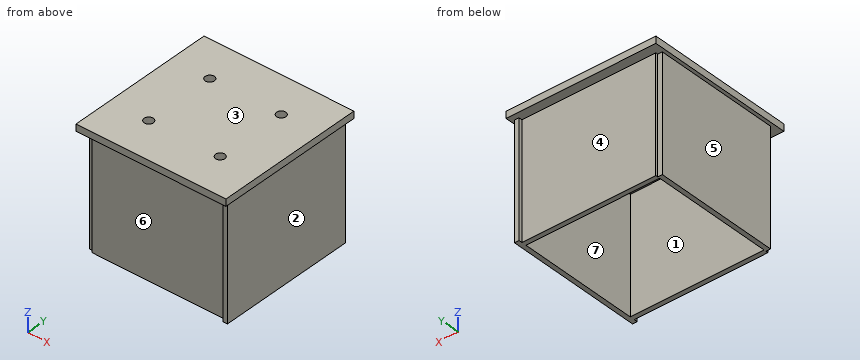
```python
from build123d import *

# Parameters (mm, degrees)
SKETCH1_W           = 65
SKETCH1_H           = 65
SKETCH1_R           = 2
BOSS_EXTRUDE1_DEPTH = 3
SKETCH4_W           = 2
SKETCH4_H           = 60
SKETCH4_H_2         = 55
BOSS_EXTRUDE3_DEPTH = 50


with BuildPart() as part:
    # Sketch1 → Boss-Extrude1 (new body)
    with BuildSketch(Plane.XY):
        Rectangle(SKETCH1_W, SKETCH1_H)
        with Locations((-15.5, 15.5)):
            Circle(SKETCH1_R, mode=Mode.SUBTRACT)
        with Locations((15.5, 15.5)):
            Circle(SKETCH1_R, mode=Mode.SUBTRACT)
        with Locations((15.5, -15.5)):
            Circle(SKETCH1_R, mode=Mode.SUBTRACT)
        with Locations((-15.5, -15.5)):
            Circle(SKETCH1_R, mode=Mode.SUBTRACT)
    extrude(amount=BOSS_EXTRUDE1_DEPTH)

    # Sketch4 → Boss-Extrude3 (add)
    with BuildSketch(Plane(origin=(0, 0, 0), x_dir=(-1, 0, 0), z_dir=(0, 0, -1))):
        with Locations((-30, 0)):
            Rectangle(SKETCH4_W, SKETCH4_H)
        Polygon((29, -26.5), (-29, -26.5), (-29, -28.5), (29, -28.5), (29, -27.5), align=None)
        with Locations((30, 0)):
            Rectangle(SKETCH4_W, SKETCH4_H_2)
        Polygon((29, 27.5), (29, 28.5), (-29, 28.5), (-29, 26.5), (29, 26.5), align=None)
    extrude(amount=BOSS_EXTRUDE3_DEPTH)


solid = part.part
```
The model under review builds one solid part; all positions refer to its coordinate system, in mm. Face numbers are marked on the shaded views. A direction names the side the tool comes from. Round coordinates to 2 decimals unless told otherwise and drop trailing zeros. Order: outer loops, then holes, each group sorted by start corner. A loop starts at its lowest first (then second) coordinate and runs counter-clockwise, first axis right, second up. Notation, with made-up numbers: (32, -25.75) -> (85, -25.75) arc R28 ccw to (85, 6.25) -> close; hole circle Ø3 at (71.5, 26.5). An arc over 180 degrees is marked (long way). One line per item, written item: value. Start each with the question number.
Q1. Take a section at D-D (x = -6). Write out the cut boundary in (y, z), and give its area (3 significant figures).
Q2. Take a section at C-C (z = -32.5). Write out the cut boundary in (x, y).
Q3. Wall thickness on line 1 (Y direction, x = 15.5, z = 2.25); line 2 (X direction, y = 15, z = 1); line 3 (X direction, y = 7, z = -25): over which ranges is each line inside the solid? List them lowest first.
Q4. Take a section at B-B (y = 15.5). Write out the cut boundary in (x, z).
Q5. Clearance check with flat-ended pins moving along their axes: pin 1 Ø5 at (y, z) = (-0.5, -15.5) entering from -X; pin 2 Ø15 at (x, z) = (-12, -32.5) entering from +Y; pin 3 Ø8 at (x, z) = (1, -22.5) entering from -Y; pin 4 Ø5 at (x, y) = (-15.5, -15.5) entering from +Z. State where each tip first meets the part, or that it passes through.
Q6. Machinability: for the marked faces 1, 2, 3 and 4, which of the approach directions +Z, -Z, +X, -X, +Y, -Y give a long, thin tool a straight path to every point of the face, cutting with its end or side? Answer none if there is none.
Q7. Take a section at A-A (x = 15.5). Write out the cut boundary in (y, z), and give its area (3 significant figures).
Q8. Mouldability with a two-part tool opening along X and no side actions: class the marked faces 5, 6 and 7 as released by +X, released by -X, zero draft, split by the parting line, or undercut.
Reported:
1. outline: (-32.5, 0) -> (-28.5, 0) -> (-28.5, -50) -> (-26.5, -50) -> (-26.5, 0) -> (26.5, 0) -> (26.5, -50) -> (28.5, -50) -> (28.5, 0) -> (32.5, 0) -> (32.5, 3) -> (-32.5, 3) -> close
1. area: 395 mm2
2. outline: (-31, -27.5) -> (-29, -27.5) -> (-29, -28.5) -> (29, -28.5) -> (29, -30) -> (31, -30) -> (31, 30) -> (29, 30) -> (29, 28.5) -> (-29, 28.5) -> (-29, 27.5) -> (-31, 27.5) -> close; hole (-29, -26.5) -> (29, -26.5) -> (29, 26.5) -> (-29, 26.5) -> close
3. line 1: y = -32.5 to -17.5, -13.5 to 13.5, 17.5 to 32.5
3. line 2: x = -32.5 to -17.44, -13.56 to 13.56, 17.44 to 32.5
3. line 3: x = -31 to -29, 29 to 31
4. outline: (-32.5, 0) -> (-31, 0) -> (-31, -50) -> (-29, -50) -> (-29, 0) -> (-17.5, 0) -> (-17.5, 3) -> (-32.5, 3) -> close; (-13.5, 0) -> (13.5, 0) -> (13.5, 3) -> (-13.5, 3) -> close; (17.5, 0) -> (29, 0) -> (29, -50) -> (31, -50) -> (31, 0) -> (32.5, 0) -> (32.5, 3) -> (17.5, 3) -> close
5. pin 1: stops at x = -31
5. pin 2: stops at y = 28.5
5. pin 3: stops at y = -28.5
5. pin 4: stops at z = 3
6. face 1: -Z
6. face 2: -Z, +X, +Y, -Y
6. face 3: +Z, +X, -X, +Y, -Y
6. face 4: -Z, -X, +Y
7. outline: (-32.5, 0) -> (-28.5, 0) -> (-28.5, -50) -> (-26.5, -50) -> (-26.5, 0) -> (-17.5, 0) -> (-17.5, 3) -> (-32.5, 3) -> close; (-13.5, 0) -> (13.5, 0) -> (13.5, 3) -> (-13.5, 3) -> close; (17.5, 0) -> (26.5, 0) -> (26.5, -50) -> (28.5, -50) -> (28.5, 0) -> (32.5, 0) -> (32.5, 3) -> (17.5, 3) -> close
7. area: 371 mm2
8. face 5: released by -X
8. face 6: zero draft
8. face 7: undercut
